```python
from build123d import *

# Parameters (mm, degrees)
SKETCH1_W          = 6.35
SKETCH1_H          = 6.096
SKETCH2_R          = 29.718
SKETCH2_R_2        = 26.543
CUT_EXTRUDE1_DEPTH = 2.032


with BuildPart() as part:
    # Sketch1 → Revolve1 (revolve)
    with BuildSketch(Plane.XY):
        Polygon((0, 25.4), (0, 18.8722), (82.55, 18.8722), (95.4532, 5.969), (101.4222, 5.969), (123.983193542, 12.0142), (123.983193542, 21.217805244), (99.371450104, 14.623108465), (88.594558569, 25.4), (12.446, 25.4), (6.35, 25.4), align=None)
        with Locations((3.175, 28.448)):
            Rectangle(SKETCH1_W, SKETCH1_H)
        Polygon((6.35, 31.496), (6.35, 25.4), (12.446, 25.4), align=None)
    revolve(axis=Axis((0, 0, 0), (-1, 0, 0)))

    # Sketch2 → Cut-Extrude1 (cut)
    with BuildSketch(Plane.ZY):
        Circle(SKETCH2_R)
        Circle(SKETCH2_R_2, mode=Mode.SUBTRACT)
    extrude(amount=-CUT_EXTRUDE1_DEPTH, mode=Mode.SUBTRACT)


solid = part.part
```
Can you work these out from the model? Positions are in its coordinate system, mm. A direction names the side the tool comes from. Give positions to 0.01 mm unless a question says otherwise; leave off trailing zeros. Loops run counter-clockwise (first coordinate to the right, second up) from the corner with the lowest first, then second, coordinate; pieces in that order, holes last. Notation, with made-up numbers: M -6,46.25 L 33,46.25 A12 cw 33,65.25 Z; hole C 40.5,-4.75 d5. An arc over 180 degrees is marked long. Use one line per item in the form item = value. Start each with the question number.
(1) I want a section at D-D, the plane x = 91. Write out the boundary of the cut face in (y, z).
(2) I want a section at C-C, the plane x = 62.5. Write out the boundary of the cut face in (y, z).
(3) Thinking about a two-plate mould opening in Z: for faces 4 (the flat face through (123.983, -9, 9)), 5 (the conical face through (106.04, 15.65, -4.93)), 6 (the cylindrical face through (41.853, -4.091, 18.423)), which applies, released by +Z, released by -Z, zero draft, split by the parting line, or undercut?
(4) I'm going to push flat-ended pins straight in: P1, Ø3, axis at x = 49, z = 5, coming from the +Y side; P2, Ø5, axis at x = 26.5, y = 17.5, coming from the -Z side; P3, Ø10, axis at x = 54.5, z = -1, coming from the +Y side. Where does each tip first touch, or does it pass through?
(5) Please list where these lines run through material, in increasing order: line 1 (Y direction, x = 1.15, z = 0); line 2 (Y direction, x = 26.5, z = 0); line 3 (Y direction, x = 49, z = 17).
(6) On a 3-axis mill with a long thin cutter (end or side, diameter ignored), from which of +Z, -Z, +X, -X, +Y, -Y can I reach the whole of each face in a straight line? I mean faces 1 (the conical face through (98.7, 8.22, -12.9)), 2 (the cylindrical face through (1, -29.01, -6.44)), 3 (the cylindrical face through (49.987, -5.506, 24.796)). Say none if no direction works.
Worked out:
q1.outline = C 0,0 d45.99; hole C 0,0 d20.84
q2.outline = C 0,0 d50.8; hole C 0,0 d37.74
q3.face_4 = zero draft
q3.face_5 = split by the parting line
q3.face_6 = undercut
q4.P1 = 25.16
q4.P2 = -20.5
q4.P3 = 25.4
q5.line_1 = -31.5 to -29.72, -26.54 to -18.87, 18.87 to 26.54, 29.72 to 31.5
q5.line_2 = -25.4 to -18.87, 18.87 to 25.4
q5.line_3 = -18.87 to -8.2, 8.2 to 18.87
q6.face_1 = none
q6.face_2 = -X
q6.face_3 = +X
